Read the model definition and answer for the solid it produces. Units are mm, in the model's axes. Face numbers are marked on the shaded views. A direction names the side the tool comes from. Round coordinates to 2 decimals unless told otherwise and drop trailing zeros. Order: outer loops, then holes, each group sorted by start corner. A loop starts at its lowest first (then second) coordinate and runs counter-clockwise, first axis right, second up. Notation, with made-up numbers: (58.5, 3.5) - (83.5, 3.5) arc R24 ccw to (83.5, 25.5) - close; hole circle Ø2 at (72.5, 54.5). An arc over 180 degrees is marked (long way). One line per question, with ' | ' between items. Start each with the question number.
1) Flat-ended cylindrical pins translate along their axes: pin 1 (0.5 mm diameter, centred on y = 21, z = -2, fed in from -X); pin 2 (2 mm diameter, centred on y = 6, z = 1, fed in from +X); pin 3 (1.5 mm diameter, centred on y = 18.5, z = -2, fed in from +X). Find the tip coordinate at first contact, or state that the pin passes through.
2) Straight lines are drawn through the part: line 1 (Z direction, x = -6.25, y = 10.5); line 2 (X direction, y = 8.5, z = -2.3); line 3 (Y direction, x = -5, z = 1.8). For each, find the intervals that lie inside material, in ascending order. Write a range as from..to.
3) The part is cut by section D-D, the plane x = 6.5. Give the vertices of the cut face in (y, z).
4) The part is cut by section C-C, the plane y = 27.5. Give the vertices of the cut face in (x, z).
5) The mould has two halves that part along Y. Classify the marked faces 1, 2, 3 and 4: pulls with the +Y half, pulls with the -Y half, needs draft (parallel to the pull), parting line crosses it, or undercut.
6) For the marked faces 5 and 6, determine the directions among +Z, -Z, +X, -X, +Y, -Y from which every point of the face is accessible in a straight line to the end or side of a thin tool.
7) The part is cut by section B-B, the plane z = 1.45. Count the separate pieces of the cut face and the enclosed holes in it, plus the area to 3 significant figures.
8) The part is cut by section A-A, the plane z = -1.85. Give the vertices of the cut face in (x, y), plus the area to 3 significant figures.
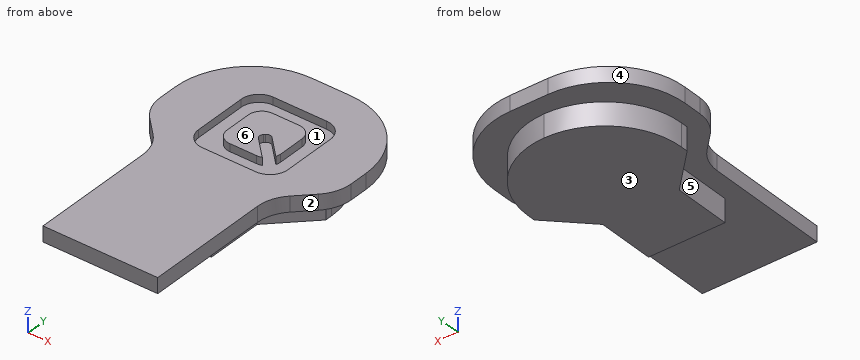
from build123d import *

# Parameters (mm, degrees)
F1_DEPTH = 2
F3_DEPTH = 3
F4_W     = 15
F4_H     = 2
F5_DEPTH = 4
F7_DEPTH = 1


with BuildPart() as f1:
    # F0 (on Top) → F1 (new body)
    with BuildSketch(Plane.XY):
        with BuildLine():
            Line((-7.5, 0), (0, 0))
            Line((0, 0), (7.5, 0))
            Line((7.5, 0), (7.5, 12.428932))
            ThreePointArc((7.5, 12.428932), (7.880602, 14.342349), (8.964466, 15.964466))
            Line((8.964466, 15.964466), (11.035534, 18.035534))
            ThreePointArc((11.035534, 18.035534), (12.119398, 19.657651), (12.5, 21.571068))
            Line((12.5, 21.571068), (12.5, 24))
            ThreePointArc((12.5, 24), (9.571068, 31.071068), (2.5, 34))
            Line((2.5, 34), (0, 34))
            Line((0, 34), (-2.5, 34))
            ThreePointArc((-2.5, 34), (-9.571068, 31.071068), (-12.5, 24))
            Line((-12.5, 24), (-12.5, 21.571068))
            ThreePointArc((-12.5, 21.571068), (-12.119398, 19.657651), (-11.035534, 18.035534))
            Line((-11.035534, 18.035534), (-8.964466, 15.964466))
            ThreePointArc((-8.964466, 15.964466), (-7.880602, 14.342349), (-7.5, 12.428932))
            Line((-7.5, 12.428932), (-7.5, 0))
        make_face()
    extrude(amount=F1_DEPTH)

    # F2 (on face) → F3 (join)
    with BuildSketch(Plane(origin=(0, 0, 0), x_dir=(1, 0, 0), z_dir=(0, 0, -1))):
        with BuildLine():
            ThreePointArc((0, -31.5), (7.071068, -28.571068), (10, -21.5))
            Line((10, -21.5), (10, -20.535534))
            Line((10, -20.535534), (5, -15.535534))
            Line((5, -15.535534), (5, -8))
            Line((5, -8), (-5, -8))
            Line((-5, -8), (-5, -15.535534))
            Line((-5, -15.535534), (-10, -20.535534))
            Line((-10, -20.535534), (-10, -21.5))
            ThreePointArc((-10, -21.5), (-7.071068, -28.571068), (0, -31.5))
        make_face()
    extrude(amount=F3_DEPTH)

    # F4 (on face) → F5 (join)
    with BuildSketch(Plane.XZ):
        with Locations((0, 1)):
            Rectangle(F4_W, F4_H)
    extrude(amount=F5_DEPTH)

    # F6 (on face) → F7 (cut)
    with BuildSketch(Plane.XY.offset(2)):
        with BuildLine():
            ThreePointArc((-5.833333, 19.535534), (-5.149916, 17.885618), (-3.5, 17.202201))
            Line((-3.5, 17.202201), (3.5, 17.202201))
            ThreePointArc((3.5, 17.202201), (5.149916, 17.885618), (5.833333, 19.535534))
            Line((5.833333, 19.535534), (5.833333, 26.535534))
            ThreePointArc((5.833333, 26.535534), (5.149916, 28.18545), (3.5, 28.868867))
            Line((3.5, 28.868867), (-3.5, 28.868867))
            ThreePointArc((-3.5, 28.868867), (-5.149916, 28.18545), (-5.833333, 26.535534))
            Line((-5.833333, 26.535534), (-5.833333, 19.535534))
        make_face()
        with BuildLine():
            Line((1.75, 19.535534), (-1.75, 19.535534))
            ThreePointArc((-1.75, 19.535534), (-2.987437, 20.048097), (-3.5, 21.285534))
            Line((-3.5, 21.285534), (-3.5, 24.785534))
            ThreePointArc((-3.5, 24.785534), (-2.987437, 26.022971), (-1.75, 26.535534))
            Line((-1.75, 26.535534), (1.75, 26.535534))
            ThreePointArc((1.75, 26.535534), (2.987437, 26.022971), (3.5, 24.785534))
            Line((3.5, 24.785534), (3.5, 21.285534))
            ThreePointArc((3.5, 21.285534), (3.46951, 20.96029), (3.379104, 20.646379))
            Line((3.379104, 20.646379), (0.907454, 23.11803))
            ThreePointArc((0.907454, 23.11803), (0.494975, 23.288884), (0.082496, 23.11803))
            Line((0.082496, 23.11803), (0, 23.035534))
            Line((0, 23.035534), (-0.082496, 22.953038))
            ThreePointArc((-0.082496, 22.953038), (-0.25335, 22.540559), (-0.082496, 22.12808))
            Line((-0.082496, 22.12808), (2.389155, 19.65643))
            ThreePointArc((2.389155, 19.65643), (2.075244, 19.566023), (1.75, 19.535534))
        make_face(mode=Mode.SUBTRACT)
    extrude(amount=-F7_DEPTH, mode=Mode.SUBTRACT)


solid = f1.part
Values:
1) pin 1: stops at x = -10 | pin 2: stops at x = 7.5 | pin 3: stops at x = 8.71
2) line 1: z = 0..2 | line 2: x = -5..5 | line 3: y = -4..17.75, 28.32..33.68
3) outline: (-4, 0) - (17.04, 0) - (17.04, -3) - (29.1, -3) - (29.1, 0) - (33.17, 0) - (33.17, 2) - (-4, 2) - close
4) outline: (-11.87, 0) - (-8, 0) - (-8, -3) - (8, -3) - (8, 0) - (11.87, 0) - (11.87, 2) - (5.62, 2) - (5.62, 1) - (-5.62, 1) - (-5.62, 2) - (-11.87, 2) - close
5) face 1: undercut | face 2: pulls with the -Y half | face 3: needs draft | face 4: pulls with the +Y half
6) face 5: -Z, -X, -Y | face 6: +Z, +X, -X, +Y, -Y
7) separate pieces: 2 | enclosed holes: 1 | area: 606 mm^2
8) outline: (-10, 20.54) - (-5, 15.54) - (-5, 8) - (5, 8) - (5, 15.54) - (10, 20.54) - (10, 21.5) arc R10 ccw to (0, 31.5) arc R10 ccw to (-10, 21.5) - close | area: 327 mm^2
